Check sheet for the modelled part. Datum: model origin and axes. Units: mm. A direction names the side the tool comes from. Round coordinates to 2 decimals unless told otherwise and drop trailing zeros. Loops run counter-clockwise (first coordinate to the right, second up) from the corner with the lowest first, then second, coordinate; pieces in that order, holes last. Notation, with made-up numbers: (15.25, 48.5) -> (61.25, 48.5) arc R28 ccw to (61.25, 86.5) -> close; hole circle Ø9 at (73, 55.25). An arc over 180 degrees is marked (long way). Use one line per item in the form item = value. Start each with the question number.
(1) Draft check along Y on faces 1 (the cylindrical face through (-10.3, -46.37, 4.93)), 2 (the cylindrical face through (-249.76, 10.99, 4.93)), 3 (the flat face through (52, 4, 0)). Enter one of: released by +Y, released by -Y, zero draft, split by the parting line, or undercut.
(2) Set-up check for faces 4 (the flat face through (52, 4, 10)), 5 (the flat face through (32.97, -121.54, 5.07)): record each of +Z, -Z, +X, -X, +Y, -Y from which the full face is reachable in a straight line by a thin tool's end or side.
(3) Material ranges on probe 1 along Y at (x, z) = (0, 7.75); probe 2 along Y at (x, z) = (142.5, 5.75); probe 3 along Y at (x, z) = (-106, 4.5), recorded low to high. Write a range as [from, to].
(4) Sectioned sample at D-D (x = 199). Record the cut outline in (y, z), and give its area (3 significant figures).
(5) Sectioned sample at B-B (y = 101). Record the cut outline in (x, z), and give its area (3 significant figures).
(6) Sectioned sample at A-A (y = 0). Record the cut outline in (x, z).
(7) Sectioned sample at C-C (z = 5.5). State how many separate pieces and enclosed holes the cut face has, and give its area (3 significant figures).
(8) Go/stop test with flat-tipped pins: pin 1 (4 mm diameter, centred on x = -72, z = 5.5, fed in from +Y); pin 2 (4 mm diameter, centred on x = 164, z = 7.5, fed in from +Y); pin 3 (1 mm diameter, centred on y = -15, z = 3, fed in from +X). Record where each tip stops, or that it passes through.
from build123d import *

# Parameters (mm, degrees)
SKETCH_R                = 250
SKETCH_R_2              = 47.5
PAD_DEPTH               = 10
POCKET_DEPTH            = 1424.355977
POCKET_MIRRORED_2_DEPTH = 1424.355977
POLARPATTERN_COUNT      = 6
SKETCH002_R             = 7
POCKET001_DEPTH         = 1424.355977
POLARPATTERN001_COUNT   = 5


with BuildPart() as part:
    # Sketch → Pad (new body)
    with BuildSketch(Plane.XY):
        Circle(SKETCH_R)
        Circle(SKETCH_R_2, mode=Mode.SUBTRACT)
    extrude(amount=PAD_DEPTH)

    # Sketch001 (on Face4 of Pad) → Pocket (cut, through all)
    with BuildSketch(Plane.XY.offset(10)):
        with BuildLine():
            Line((22.514747, 83.000519), (43.720498, 161.175426))
            ThreePointArc((43.720498, 161.175426), (22.053387, 165.537452), (0, 167))
            Line((0, 86), (0, 167))
            ThreePointArc((22.514747, 83.000519), (11.356834, 85.246832), (0, 86))
        make_face()
    pocket = extrude(amount=-POCKET_DEPTH, mode=Mode.SUBTRACT)

    # Sketch001 Mirrored 2 → Pocket Mirrored 2 (cut, through all)
    with BuildSketch(Plane(origin=(0, 0, 10), x_dir=(-1, 0, 0), z_dir=(0, 0, -1))):
        with BuildLine():
            Line((22.514747, 83.000519), (43.720498, 161.175426))
            ThreePointArc((43.720498, 161.175426), (22.053387, 165.537452), (0, 167))
            Line((0, 86), (0, 167))
            ThreePointArc((22.514747, 83.000519), (11.356834, 85.246832), (0, 86))
        make_face()
    pocket_mirrored_2 = extrude(amount=POCKET_MIRRORED_2_DEPTH, mode=Mode.SUBTRACT)

    # PolarPattern: Pocket, Pocket Mirrored 2 ×6 about axis
    polarpattern_axis = Axis((0, 0, 10), (0, 0, 1))
    for i in range(1, POLARPATTERN_COUNT):
        add(pocket.rotate(polarpattern_axis, i * 360 / POLARPATTERN_COUNT), mode=Mode.SUBTRACT)
        add(pocket_mirrored_2.rotate(polarpattern_axis, i * 360 / POLARPATTERN_COUNT), mode=Mode.SUBTRACT)

    # Sketch002 (on Face4 of Pad) → Pocket001 (cut, through all)
    with BuildSketch(Plane.XY.offset(10)):
        with Locations((0, 65)):
            Circle(SKETCH002_R)
    pocket001 = extrude(amount=-POCKET001_DEPTH, mode=Mode.SUBTRACT)

    # PolarPattern001: Pocket001 ×5 about axis
    polarpattern001_axis = Axis((0, 0, 10), (0, 0, 1))
    for i in range(1, POLARPATTERN001_COUNT):
        add(pocket001.rotate(polarpattern001_axis, i * 360 / POLARPATTERN001_COUNT), mode=Mode.SUBTRACT)


solid = part.part
Checks:
q1.face_1 = undercut
q1.face_2 = split by the parting line
q1.face_3 = zero draft
q2.face_4 = +Z, +X, -X, +Y, -Y
q2.face_5 = +Z, -Z
q3.probe_1 = [-250, -167], [-86, -47.5], [47.5, 58], [72, 86], [167, 250]
q3.probe_2 = [-205.41, -87.08], [-37.71, 37.71], [87.08, 205.41]
q3.probe_3 = [-226.42, -106.66], [-28.05, 28.05], [106.66, 226.42]
q4.outline = (-151.32, 0) -> (151.32, 0) -> (151.32, 10) -> (-151.32, 10) -> close
q4.area = 3,030 mm2
q5.outline = (-228.69, 0) -> (-133, 0) -> (-133, 10) -> (-228.69, 10) -> close; (-100.38, 0) -> (-27.4, 0) -> (-27.4, 10) -> (-100.38, 10) -> close; (27.4, 0) -> (100.38, 0) -> (100.38, 10) -> (27.4, 10) -> close; (133, 0) -> (228.69, 0) -> (228.69, 10) -> (133, 10) -> close
q5.area = 3,370 mm2
q6.outline = (-250, 0) -> (-47.5, 0) -> (-47.5, 10) -> (-250, 10) -> close; (47.5, 0) -> (250, 0) -> (250, 10) -> (47.5, 10) -> close
q7.separate_pieces = 1
q7.enclosed_holes = 12
q7.area = 156,000 mm2
q8.pin_1 = 240
q8.pin_2 = 190.41
q8.pin_3 = 249.58
